from build123d import *

# Parameters (mm, degrees)
SKETCH1_W           = 75
SKETCH1_H           = 105
BOSS_EXTRUDE1_DEPTH = 9
SKETCH2_R           = 9
SKETCH2_R_2         = 2
SKETCH2_R_3         = 5.1
SKETCH2_R_4         = 1.825
CUT_EXTRUDE1_DEPTH  = 9
CHAMFER1_SIZE       = 50
FILLET1_R           = 15


with BuildPart() as part:
    # Sketch1 → Boss-Extrude1 (new body)
    with BuildSketch(Plane(origin=(0, 0, 0), x_dir=(1, 0, 0), z_dir=(0, 1, 0))):
        with Locations((37.5, 52.5)):
            Rectangle(SKETCH1_W, SKETCH1_H)
    extrude(amount=BOSS_EXTRUDE1_DEPTH)

    # Sketch2 → Cut-Extrude1 (cut)
    with BuildSketch(Plane(origin=(0, 9, 0), x_dir=(1, 0, 0), z_dir=(0, 1, 0))):
        with Locations((15, 15)):
            Circle(SKETCH2_R)
        with Locations((15, 50)):
            Circle(SKETCH2_R_2)
        with Locations((60, 15)):
            Circle(SKETCH2_R_3)
        with Locations((60, 23)):
            Circle(SKETCH2_R_4)
        with Locations((60, 7)):
            Circle(SKETCH2_R_4)
        with Locations((68, 15)):
            Circle(SKETCH2_R_4)
        with Locations((52, 15)):
            Circle(SKETCH2_R_4)
        with Locations((60, 90)):
            Circle(SKETCH2_R_3)
        with Locations((60, 98)):
            Circle(SKETCH2_R_4)
        with Locations((60, 82)):
            Circle(SKETCH2_R_4)
        with Locations((68, 90)):
            Circle(SKETCH2_R_4)
        with Locations((52, 90)):
            Circle(SKETCH2_R_4)
    extrude(amount=-CUT_EXTRUDE1_DEPTH, mode=Mode.SUBTRACT)

    # Chamfer1
    chamfer1_edges = [part.edges().sort_by_distance(p)[0] for p in [
        (0, 4.5, -105),
    ]]
    chamfer(chamfer1_edges, length=CHAMFER1_SIZE)

    # Fillet1
    fillet1_edges = [part.edges().sort_by_distance(p)[0] for p in [
        (0, 4.5, -55),
        (50, 4.5, -105),
        (75, 4.5, -105),
        (75, 4.5, 0),
        (0, 4.5, 0),
    ]]
    fillet(fillet1_edges, radius=FILLET1_R)


solid = part.part
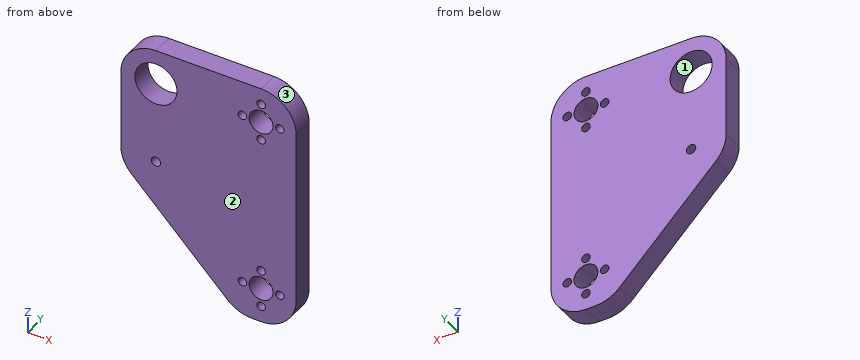
Geometry check sheet. Reference: the model listing, model coordinates, mm. Face numbers are marked on the shaded views. Give positions to 0.01 mm unless a question says otherwise; leave off trailing zeros. Loops run counter-clockwise (first coordinate to the right, second up) from the corner with the lowest first, then second, coordinate; pieces in that order, holes last.
(1) Depth check by flat-ended pin: pin 1 Ø3 at (x, z) = (68, -15) entering from +Y; pin 2 Ø4 at (y, z) = (2.5, -57) entering from -X. Enter the tip coordinate at first touch or a pass-through.
From the geometry:
pin 1: passes through
pin 2: stops at x = 1.35
(2) Thickness scan on L1, parallel to X at y = 6.5, z = -90 (3 decimals); L2, parallel to Z at x = 52, y = 4 (3 decimals); L3, parallel to Z at x = 68, y = 2.5 (3 decimals). Record the ranges inside material, lowest first.
From the geometry:
L1: x = 35 to 50.175, 53.825 to 54.9, 65.1 to 66.175, 69.825 to 75
L2: z = -104.396 to -91.825, -88.175 to -16.825, -13.175 to 0
L3: z = -102.689 to -91.825, -88.175 to -16.825, -13.175 to -2.311
(3) Section check D-D on z = -76. Record the cut outline in (x, y).
From the geometry:
outline: (21, 0) - (75, 0) - (75, 9) - (21, 9) - close
(4) Release check for a two-part mould opening along X. For the marked faces 1, 2 and 3 record: released by +X, released by -X, zero draft, split by the parting line, or undercut.
From the geometry:
face 1: undercut
face 2: zero draft
face 3: released by +X
(5) Section check B-B on x = 21. Record the cut outline in (y, z).
From the geometry:
outline: (0, -76) - (9, -76) - (9, -21.71) - (0, -21.71) - close; (0, -8.29) - (9, -8.29) - (9, 0) - (0, 0) - close
(6) Section check A-A on y = 3.25. Count the separate pieces of the cut face and the enclosed holes in it, then the cut area to 3 significant figures.
From the geometry:
separate pieces: 1
enclosed holes: 12
area: 5,960 mm2
(7) Section check C-C on z = -50. Record the cut outline in (x, y), then the cut area to 3 significant figures.
From the geometry:
outline: (0.05, 0) - (13, 0) - (13, 9) - (0.05, 9) - close; (17, 0) - (75, 0) - (75, 9) - (17, 9) - close
area: 639 mm2
